```python
from build123d import *

# Parameters (mm, degrees)
BOSS_EXTRUDE1_DEPTH = 2
SKETCH2_W           = 40
SKETCH2_H           = 50
BOSS_EXTRUDE2_DEPTH = 2
BOSS_EXTRUDE3_DEPTH = 4
SKETCH5_R           = 4
CUT_EXTRUDE2_DEPTH  = 44


with BuildPart() as part:
    # Sketch1 → Boss-Extrude1 (new body)
    with BuildSketch(Plane(origin=(0, 0, 0), x_dir=(0, 0, -1), z_dir=(1, 0, 0))):
        with BuildLine():
            Line((-13.843343537, 2.088501785), (-5.545666183, 57.088501785))
            Line((-5.545666183, 57.088501785), (-5.545666183, 62.088501785))
            Line((-5.545666183, 62.088501785), (44.454333817, 62.088501785))
            Line((44.454333817, 62.088501785), (44.454333817, 49.719071836))
            ThreePointArc((44.454333817, 49.719071836), (44.244333611, 48.145571793), (43.629033022, 46.682216861))
            Line((43.629033022, 46.682216861), (12.074298145, -7.085994941))
            ThreePointArc((12.074298145, -7.085994941), (-4.671747847, -13.197529013), (-13.843343537, 2.088501785))
        make_face()
    extrude(amount=-BOSS_EXTRUDE1_DEPTH)


with BuildPart() as body_2:
    # Mirror1: mirrored copy
    add(part.part.mirror(Plane(origin=(-20, 0, 0), x_dir=(0, 0, 1), z_dir=(1, 0, 0))))


with BuildPart() as part_1:
    add(part.part)

    add(body_2.part)  # Boss-Extrude2 merges body 2
    # Sketch2 → Boss-Extrude2 (add)
    with BuildSketch(Plane(origin=(0, 62.088501785, 0), x_dir=(1, 0, 0), z_dir=(0, 1, 0))):
        with Locations((-20, 19.454333817)):
            Rectangle(SKETCH2_W, SKETCH2_H)
    extrude(amount=-BOSS_EXTRUDE2_DEPTH)

    # Sketch3 → Boss-Extrude3 (add)
    with BuildSketch(Plane(origin=(0, 62.088501785, 0), x_dir=(1, 0, 0), z_dir=(0, 1, 0))):
        with BuildLine():
            Line((-18, 13.59419702), (-9.643842411, 29.454333817))
            ThreePointArc((-9.643842411, 29.454333817), (-20, 11.392155991), (-30.356157589, 29.454333817))
            Line((-30.356157589, 29.454333817), (-22, 13.59419702))
            ThreePointArc((-22, 13.59419702), (-20, 13.392155991), (-18, 13.59419702))
        make_face()
    extrude(amount=-BOSS_EXTRUDE3_DEPTH)

    # Sketch5 → Cut-Extrude2 (cut)
    with BuildSketch(Plane(origin=(0, 0, 0), x_dir=(0, 0, -1), z_dir=(1, 0, 0))):
        with Locations(Location((0, 0, 0), (0, 0, 180))):
            Circle(SKETCH5_R)
    extrude(amount=-CUT_EXTRUDE2_DEPTH, mode=Mode.SUBTRACT)


solid = part_1.part
```
The listing builds one solid part. Answer for the finished solid, in the listing's coordinates (mm). A direction names the side the tool comes from. Coordinates: 2 decimals unless noted, no trailing zeros. Order: outer loops, then holes, each group sorted by start corner. A loop starts at its lowest first (then second) coordinate and runs counter-clockwise, first axis right, second up. Notation, with made-up numbers: M 25.25,-20 L 71.25,-20 A10 ccw 71.25,-2 Z; hole C 37.5,30.5 d3. An arc over 180 degrees is marked long. Answer as a JSON object with one key per item and string values. Group by question number.
1. Section A-A on z = 0 is taken. Write down the section's boundary in (x, y), then the cut area to 3 significant figures.
2. Straight lines are drawn through the part: line 1 (Y direction, x = -1, z = 0); line 2 (X direction, y = 53.5, z = -22); line 3 (Y direction, x = -35, z = -41). For each, find the intervals that lie inside material, in ascending order.
3. Section D-D on y = 32.5 is taken. Write down the section's boundary in (x, z), then the cut area to 3 significant figures.
4. Flat-ended cylindrical pins translate along their axes: P1, Ø4, axis at x = -29, z = -10, coming from the -Y side; P2, Ø6.5, axis at y = 0, z = 0, coming from the -X side; P3, Ø5.5, axis at x = -19.5, y = 59, coming from the +Z side; P4, Ø1.5, axis at x = -16, z = -17, coming from the -Y side. Find the tip coordinate at first contact, or state that the pin passes through.
5. Section C-C on x = -20 is taken. Write down the section's boundary in (y, z), then the cut area to 3 significant figures.
6. Determine the mould class of faces 1 (the flat face through (-39.01, 20.17, -28.07)), 2 (the flat face through (-0.986, 29.204, 9.753)), 3 (the cylindrical face through (-38.986, 3.905, -0.867)), 4 (the cylindrical face through (-0.986, 3.905, -0.867)) for opening direction Z: released by +Z, released by -Z, zero draft, split by the parting line, or undercut.
7. Section B-B on y = 1 is taken. Write down the section's boundary in (x, z).
8. A tool of negligible diameter and unlimited length cuts with its end or side. For faces 5 (the cylindrical face through (-39.01, 48.17, -44.25)), 6 (the flat face through (-26.24, 59.1, -21.64)), 7 (the flat face through (-20, 60.089, -20)), 8 (the flat face through (-20, 62.089, -20)), 9 (the flat face through (-2, 32, -9)), from which of +Z, -Z, +X, -X, +Y, -Y can it reach the whole face along a straight path? Write none if from no direction.
Values follow:
{
 "1": {"outline": "M -40,-14 L -38,-14 L -38,-4 L -40,-4 Z; M -40,4 L -38,4 L -38,60.09 L -2,60.09 L -2,4 L 0,4 L 0,62.09 L -40,62.09 Z; M -2,-14 L 0,-14 L 0,-4 L -2,-4 Z", "area": "344 mm2"},
 "2": {"line 1": "-14 to -4, 4 to 62.09", "line 2": "-40 to -38, -2 to 0", "line 3": "60.09 to 62.09"},
 "3": {"outline": "M -40,-35.31 L -38,-35.31 L -38,9.26 L -40,9.26 Z; M -2,-35.31 L 0,-35.31 L 0,9.26 L -2,9.26 Z", "area": "178 mm2"},
 "4": {"P1": "y = 60.09", "P2": "through", "P3": "z = 5.55", "P4": "y = 58.09"},
 "5": {"outline": "M 58.09,-13.39 L 60.09,-13.39 L 60.09,-44.45 L 62.09,-44.45 L 62.09,5.55 L 60.09,5.55 L 60.09,-11.39 L 58.09,-11.39 Z", "area": "104 mm2"},
 "6": {"face 1": "released by -Z", "face 2": "released by +Z", "face 3": "undercut", "face 4": "undercut"},
 "7": {"outline": "M -40,-16.82 L -38,-16.82 L -38,-3.87 L -40,-3.87 Z; M -40,3.87 L -38,3.87 L -38,13.96 L -40,13.96 Z; M -2,-16.82 L 0,-16.82 L 0,-3.87 L -2,-3.87 Z; M -2,3.87 L 0,3.87 L 0,13.96 L -2,13.96 Z"},
 "8": {"face 5": "-Z, +X, -X, -Y", "face 6": "-Z, -Y", "face 7": "-Y", "face 8": "+Z, -Z, +X, -X, +Y", "face 9": "+Z, -Z, -Y"}
}
